Read the model definition and answer for the solid it produces. Units are mm, in the model's axes. A direction names the side the tool comes from. Give positions to 0.01 mm unless a question says otherwise; leave off trailing zeros. Write each loop counter-clockwise with the first axis right and the second up, starting at its lowest first coordinate (ties: lowest second). Pieces come first, ordered by that corner, then holes.
```python
from build123d import *

# Parameters (mm, degrees)
F0_W     = 20
F0_H     = 40
F1_DEPTH = 100
F2_R     = 5
F3_DEPTH = 25
F4_R     = 5
F5_DEPTH = 25


with BuildPart() as f1:
    # F0 (on Top) → F1 (new body)
    with BuildSketch(Plane.XY):
        Rectangle(F0_W, F0_H)
    extrude(amount=F1_DEPTH)

    # F2 (on face) → F3 (cut)
    with BuildSketch(Plane.XY.offset(100)):
        Circle(F2_R)
    extrude(amount=-F3_DEPTH, mode=Mode.SUBTRACT)

    # F4 (on face) → F5 (cut)
    with BuildSketch(Plane(origin=(0, 0, 0), x_dir=(1, 0, 0), z_dir=(0, 0, -1))):
        Circle(F4_R)
    extrude(amount=-F5_DEPTH, mode=Mode.SUBTRACT)


solid = f1.part
```
Item 1: Section B-B (x = 0) is taken. Write down the section's boundary in (y, z).
Result set:
outline: (-20, 0) - (-5, 0) - (-5, 25) - (5, 25) - (5, 0) - (20, 0) - (20, 100) - (5, 100) - (5, 75) - (-5, 75) - (-5, 100) - (-20, 100) - close
Item 2: Section C-C (z = 13) is taken. Write down the section's boundary in (x, y), and give its area (3 significant figures).
Result set:
outline: (-10, -20) - (10, -20) - (10, 20) - (-10, 20) - close; hole circle Ø10 at (0, 0)
area: 721 mm2
Item 3: Which of the six approach directions +Z, -Z, +X, -X, +Y, -Y give full straight-line access (tool end or side, diameter ignored) to faces 1 (the flat face through (2, 5, 0)), 2 (the flat face through (0, 0, 25)), 3 (the flat face through (0, 0, 75))?
Result set:
face 1: -Z, +X, -X, +Y, -Y
face 2: -Z
face 3: +Z
Item 4: Find the intervals of material crossed by line 1 along Y through (x, z) = (0, 86.5); line 2 along X through (y, z) = (-1, 7.5); line 3 along Z through (x, y) = (-1.5, -2.5), in increasing order.
Result set:
line 1: y = -20 to -5, 5 to 20
line 2: x = -10 to -4.9, 4.9 to 10
line 3: z = 25 to 75
Item 5: This flat-tipped pin is pushed along its axis until it touches: pin 1 Ø3 at (x, y) = (-1.5, -2.5) entering from -Z. Where does it stop, or does it pass through?
Result set:
pin 1: stops at z = 25
Item 6: Section A-A (y = 0) is taken. Write down the section's boundary in (x, z), and give its area (3 significant figures).
Result set:
outline: (-10, 0) - (-5, 0) - (-5, 25) - (5, 25) - (5, 0) - (10, 0) - (10, 100) - (5, 100) - (5, 75) - (-5, 75) - (-5, 100) - (-10, 100) - close
area: 1,500 mm2
Item 7: Determine the mould class of faces 4 (the flat face through (10, 0, 49)), 5 (the cylindrical face through (-1.08, 4.88, 12.32)), 6 (the flat face through (2, 5, 100)) for opening direction X: pulls with the +X half, pulls with the -X half, needs draft (parallel to the pull), parting line crosses it, or undercut.
Result set:
face 4: pulls with the +X half
face 5: undercut
face 6: needs draft
